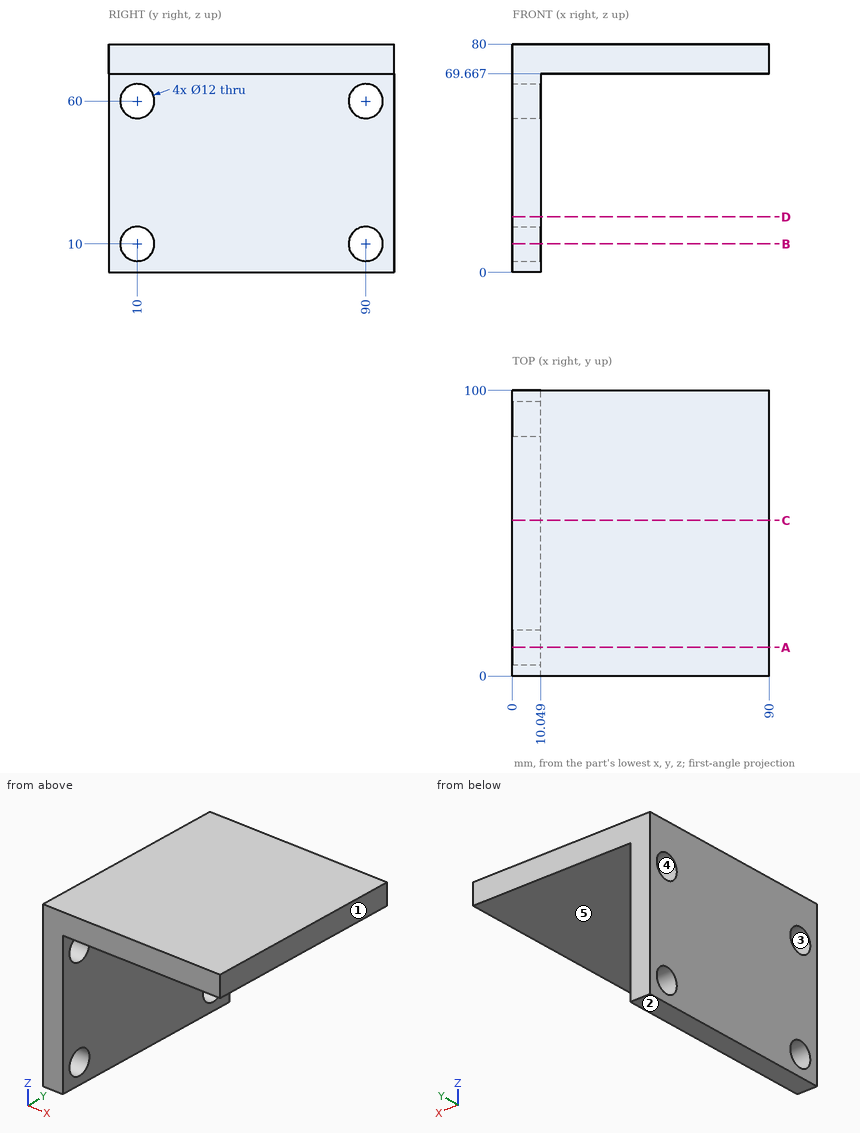
Design review of the part shown in the three views and the two pictorial views. Dimensions are in mm from the part's minimum x, y and z. A direction names the side the tool comes from. Give positions to 0.01 mm unless a question says otherwise; leave off trailing zeros. Write each loop counter-clockwise with the first axis right and the second up, starting at its lowest first coordinate (ties: lowest second). Pieces come first, ordered by that corner, then holes. Notation, with made-up numbers: M 9.25,68 L 47.25,68 A11 ccw 47.25,78 Z; hole C 63,69.25 d4. An arc over 180 degrees is marked long. Return JSON: item names as keys, results as strings. Group by question number.
Item 1: Tool access review of the marked faces 4 and 5: name each direction out of +Z, -Z, +X, -X, +Y, -Y from which nothing blocks a thin tool from reaching the whole face with its end or side.
Item 2: Take a section at A-A (y = 10). Give the boundary of the cut face in (x, z).
Item 3: The part is to be moulded in two halves that separate along Z. For the marked faces 1, 2 and 3, say which applies: pulls with the +Z half, pulls with the -Z half, needs draft (parallel to the pull), parting line crosses it, or undercut.
Item 4: Wall thickness on line 1 along Z through (x, y) = (5.25, 10); line 2 along Z through (x, y) = (8, 87.5) (1 decimal); line 3 along Z through (x, y) = (23.5, 24): over which ranges is each line inside the solid? List them lowest first.
Item 5: Take a section at B-B (z = 10). Give the boundary of the cut face in (x, y), plus the area to 3 significant figures.
Item 6: Take a section at D-D (z = 19.5). Give the boundary of the cut face in (x, y), plus the area to 4 significant figures.
Item 7: Clearance check with flat-ended pins moving along their axes: pin 1 Ø6 at (x, y) = (50.5, 43) entering from -Z; pin 2 Ø21 at (y, z) = (52, 20) entering from +X. State where each tip first meets the part, or that it passes through.
Item 8: Take a section at C-C (y = 54.5). Give the boundary of the cut face in (x, z), plus the area to 3 significant figures.
Return value:
{
 "1": {"face 4": "+X, -X", "face 5": "-Z, +X, +Y, -Y"},
 "2": {"outline": "M 0,0 L 10.05,0 L 10.05,4 L 0,4 Z; M 0,16 L 10.05,16 L 10.05,54 L 0,54 Z; M 0,66 L 10.05,66 L 10.05,69.67 L 90,69.67 L 90,80 L 0,80 Z"},
 "3": {"face 1": "needs draft", "face 2": "pulls with the -Z half", "face 3": "undercut"},
 "4": {"line 1": "z = 0 to 4, 16 to 54, 66 to 80", "line 2": "z = 0 to 4.5, 15.5 to 54.5, 65.5 to 80", "line 3": "z = 69.67 to 80"},
 "5": {"outline": "M 0,0 L 10.05,0 L 10.05,4 L 0,4 Z; M 0,16 L 10.05,16 L 10.05,84 L 0,84 Z; M 0,96 L 10.05,96 L 10.05,100 L 0,100 Z", "area": "764 mm2"},
 "6": {"outline": "M 0,0 L 10.05,0 L 10.05,100 L 0,100 Z", "area": "1,005 mm2"},
 "7": {"pin 1": "stops at z = 69.67", "pin 2": "stops at x = 10.05"},
 "8": {"outline": "M 0,0 L 10.05,0 L 10.05,69.67 L 90,69.67 L 90,80 L 0,80 Z", "area": "1,630 mm2"}
}
